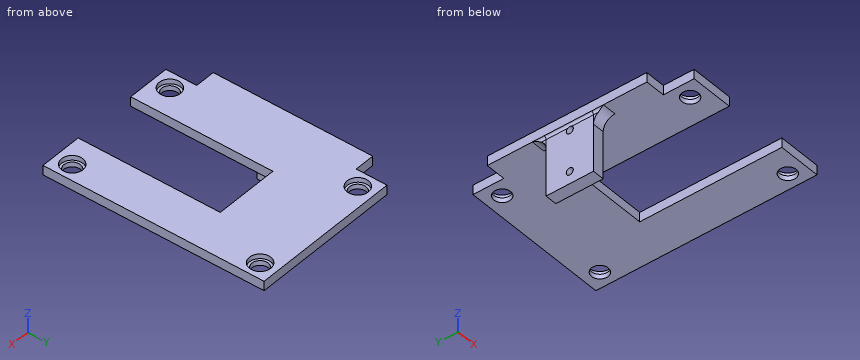
from build123d import *

# Parameters (mm, degrees)
CROQUIS1_W                 = 64.38677758
CROQUIS1_H                 = 93.345
SALIENTE_EXTRUIR1_DEPTH    = 4
CROQUIS2_W                 = 27.12677758
CROQUIS2_H                 = 60
CORTAR_EXTRUIR1_DEPTH      = 114.467819897
CROQUIS5_R                 = 4.5
CORTAR_EXTRUIR3_DEPTH      = 2
CROQUIS6_R                 = 3.5
CORTAR_EXTRUIR4_DEPTH      = 114.414929141
CROQUIS7_W                 = 8
CROQUIS7_H                 = 67.345
SALIENTE_EXTRUIR4_DEPTH    = 4
CROQUIS8_W                 = 26.63
CROQUIS8_H                 = 67.345
SALIENTE_EXTRUIR5_DEPTH    = 2
CROQUIS9_W                 = 0.5
CROQUIS9_H                 = 93.345
CROQUIS9_H_2               = 13
CORTAR_EXTRUIR5_DEPTH      = 13
CROQUIS10_W                = 5
CROQUIS10_H                = 20
SALIENTE_EXTRUIR6_DEPTH    = 25
REDONDEO1_R                = 1
REDONDEO2_START            = -8.0000001
REDONDEO2_DEPTH            = 6.0000001
REDONDEO2_START_2          = 13
REDONDEO2_2_DEPTH          = 67.345
CORTAR_EXTRUIR6_DEPTH      = 120.846669794
CORTAR_EXTRUIR6_DEPTH_BACK = 120.846669794
CROQUIS11_R                = 1.5


with BuildPart() as part:
    # Croquis1 → Saliente-Extruir1 (new body)
    with BuildSketch(Plane.XY):
        with Locations((32.19338879, 46.6725)):
            Rectangle(CROQUIS1_W, CROQUIS1_H)
    extrude(amount=SALIENTE_EXTRUIR1_DEPTH)

    # Croquis2 → Cortar-Extruir1 (cut, through all)
    with BuildSketch(Plane.XY.offset(4)):
        with Locations((32.19338879, 30)):
            Rectangle(CROQUIS2_W, CROQUIS2_H)
    extrude(amount=-CORTAR_EXTRUIR1_DEPTH, mode=Mode.SUBTRACT)

    # Croquis5 → Cortar-Extruir3 (cut)
    with BuildSketch(Plane.XY.offset(4)):
        with Locations((57.38677758, 86.345)):
            Circle(CROQUIS5_R)
        with Locations((7, 86.345)):
            Circle(CROQUIS5_R)
        with Locations((57.38677758, 7)):
            Circle(CROQUIS5_R)
        with Locations((7, 7)):
            Circle(CROQUIS5_R)
    extrude(amount=-CORTAR_EXTRUIR3_DEPTH, mode=Mode.SUBTRACT)

    # Croquis6 → Cortar-Extruir4 (cut, through all)
    with BuildSketch(Plane.XY.offset(2)):
        with Locations((7, 86.345)):
            Circle(CROQUIS6_R)
        with Locations((57.38677758, 86.345)):
            Circle(CROQUIS6_R)
        with Locations((57.38677758, 7)):
            Circle(CROQUIS6_R)
        with Locations((7, 7)):
            Circle(CROQUIS6_R)
    extrude(amount=-CORTAR_EXTRUIR4_DEPTH, mode=Mode.SUBTRACT)

    # Croquis7 → Saliente-Extruir4 (add, through all)
    with BuildSketch(Plane(origin=(0, 0, 0), x_dir=(-1, 0, 0), z_dir=(0, 0, -1))):
        with Locations((4, 46.6725)):
            Rectangle(CROQUIS7_W, CROQUIS7_H)
    extrude(amount=-SALIENTE_EXTRUIR4_DEPTH)

    # Croquis8 → Saliente-Extruir5 (add)
    with BuildSketch(Plane(origin=(0, 0, 0), x_dir=(-1, 0, 0), z_dir=(0, 0, -1))):
        with Locations((-5.315, 46.6725)):
            Rectangle(CROQUIS8_W, CROQUIS8_H)
    extrude(amount=-SALIENTE_EXTRUIR5_DEPTH)

    # Croquis9 → Cortar-Extruir5 (cut)
    with BuildSketch(Plane(origin=(0, 0, 0), x_dir=(-1, 0, 0), z_dir=(0, 0, -1))):
        with Locations((-64.13677758, 46.6725)):
            Rectangle(CROQUIS9_W, CROQUIS9_H)
        with Locations((-0.25, 86.845)):
            Rectangle(CROQUIS9_W, CROQUIS9_H_2)
        with Locations((-0.25, 6.5)):
            Rectangle(CROQUIS9_W, CROQUIS9_H_2)
    extrude(amount=-CORTAR_EXTRUIR5_DEPTH, mode=Mode.SUBTRACT)

    # Croquis10 → Saliente-Extruir6 (add)
    with BuildSketch(Plane(origin=(0, 0, 0), x_dir=(-1, 0, 0), z_dir=(0, 0, -1))):
        with Locations((4.5, 46.345)):
            Rectangle(CROQUIS10_W, CROQUIS10_H)
    extrude(amount=SALIENTE_EXTRUIR6_DEPTH)

    # Redondeo1
    redondeo1_edges = [part.edges().sort_by_distance(p)[0] for p in [
        (-7, 46.345, 0),
    ]]
    fillet(redondeo1_edges, radius=REDONDEO1_R - 0.0001)  # a hair under: the kernel refuses the full size

    # Redondeo2: read off the stored shape, not the designer's step
    # Redondeo2 outline → Redondeo2 (add)
    with BuildSketch(Plane.YZ.offset(REDONDEO2_START)):
        with BuildLine():
            Line((56.345, 0), (56.345, -5))
            ThreePointArc((56.345, -5), (57.809466094, -1.464466094), (61.345, 0))
            Line((61.345, 0), (56.345, 0))
        make_face()
        with BuildLine():
            Line((36.345, -5), (36.345, 0))
            Line((36.345, 0), (31.345, 0))
            ThreePointArc((31.345, 0), (34.880533906, -1.464466094), (36.345, -5))
        make_face()
    extrude(amount=REDONDEO2_DEPTH)

    # Redondeo2 2 outline → Redondeo2 2 (cut)
    with BuildSketch(Plane(origin=(0, 0, 0), x_dir=(1, 0, 0), z_dir=(0, 1, 0)).offset(REDONDEO2_START_2)):
        with BuildLine():
            ThreePointArc((-8, 0), (-7.292893219, 0.292893219), (-7, 1))
            Line((-7, 1), (-6.999999997, 6))
            Line((-6.999999997, 6), (-8, 6))
            Line((-8, 6), (-8, 0))
        make_face()
    extrude(amount=REDONDEO2_2_DEPTH, mode=Mode.SUBTRACT)

    # Croquis11 → Cortar-Extruir6 (cut, two sides: drawn at the far end of the back side and taken through both)
    with BuildSketch(Plane.ZY.offset(7).offset(-CORTAR_EXTRUIR6_DEPTH_BACK)):
        with Locations(Location((-19.75, 46.345, 0), (0, 0, 270))):
            Circle(CROQUIS11_R)
        with Locations(Location((-2.25, 46.345, 0), (0, 0, 270))):
            Circle(CROQUIS11_R)
    extrude(amount=CORTAR_EXTRUIR6_DEPTH + CORTAR_EXTRUIR6_DEPTH_BACK, mode=Mode.SUBTRACT)


solid = part.part
Geometry: final body of the model. Coordinates: model frame, mm. Coordinates: 2 decimals unless noted, no trailing zeros. Loops run counter-clockwise (first coordinate to the right, second up) from the corner with the lowest first, then second, coordinate; pieces in that order, holes last. Notation, with made-up numbers: M -16,6.25 L 15,6.25 A23 ccw 15,23.25 Z; hole C 66,47.5 d11. An arc over 180 degrees is marked long. One line per item, written item: value. Start each with the question number.
1) Cut plane A-A (y = 7). Return loops of the section in (x, z).
2) Cut plane D-D (y = 51). Return loops of the section in (x, z).
3) Material intervals for L1, parallel to X at y = 28.5, z = 1.5; L2, parallel to X at y = 46, z = -11.75; L3, parallel to Z at x = 47, y = 5, sorted ascending. Write a range as from..to.
4) Cut plane B-B (z = -19.75). Return loops of the section in (x, y) (3 decimals), then the cut area to 3 significant figures.
5) Pin query (flat end, axial travel): P1, Ø3, axis at x = -4.5, z = 2.5, coming from the -Y side; P2, Ø2, axis at x = -5.5, z = 2, coming from the +Y side (3 decimals); P3, Ø2, axis at y = 88, z = 2, coming from the -X side. Return the tip coordinate at first contact, or that it passes through.
6) Cut plane C-C (x = 7). Return loops of the section in (y, z) (3 decimals).
Evaluation:
1. outline: M 0.5,0 L 3.5,0 L 3.5,2 L 2.5,2 L 2.5,4 L 0.5,4 Z; M 10.5,0 L 18.63,0 L 18.63,4 L 11.5,4 L 11.5,2 L 10.5,2 Z; M 45.76,0 L 53.89,0 L 53.89,2 L 52.89,2 L 52.89,4 L 45.76,4 Z; M 60.89,0 L 63.89,0 L 63.89,4 L 61.89,4 L 61.89,2 L 60.89,2 Z
2. outline: M -8,0 A1 cw -7,-1 L -7,-25 L -2,-25 L -2,0 L 18.63,0 L 18.63,4 L -8,4 Z; M 45.76,0 L 63.89,0 L 63.89,4 L 45.76,4 Z
3. L1: -8..18.63, 45.76..63.89
3. L2: -7..-2
3. L3: 0..4
4. outline: M -7,36.345 L -2,36.345 L -2,44.845 L -7,44.845 Z; M -7,47.845 L -2,47.845 L -2,56.345 L -7,56.345 Z
4. area: 85.0 mm^2
5. P1: y = 13
5. P2: y = 80.345
5. P3: x = 0.5
6. outline: M 0,0 L 3.5,0 L 3.5,2 L 2.5,2 L 2.5,4 L 0,4 Z; M 10.5,0 L 82.845,0 L 82.845,2 L 81.845,2 L 81.845,4 L 11.5,4 L 11.5,2 L 10.5,2 Z; M 89.845,0 L 93.345,0 L 93.345,4 L 90.845,4 L 90.845,2 L 89.845,2 Z
